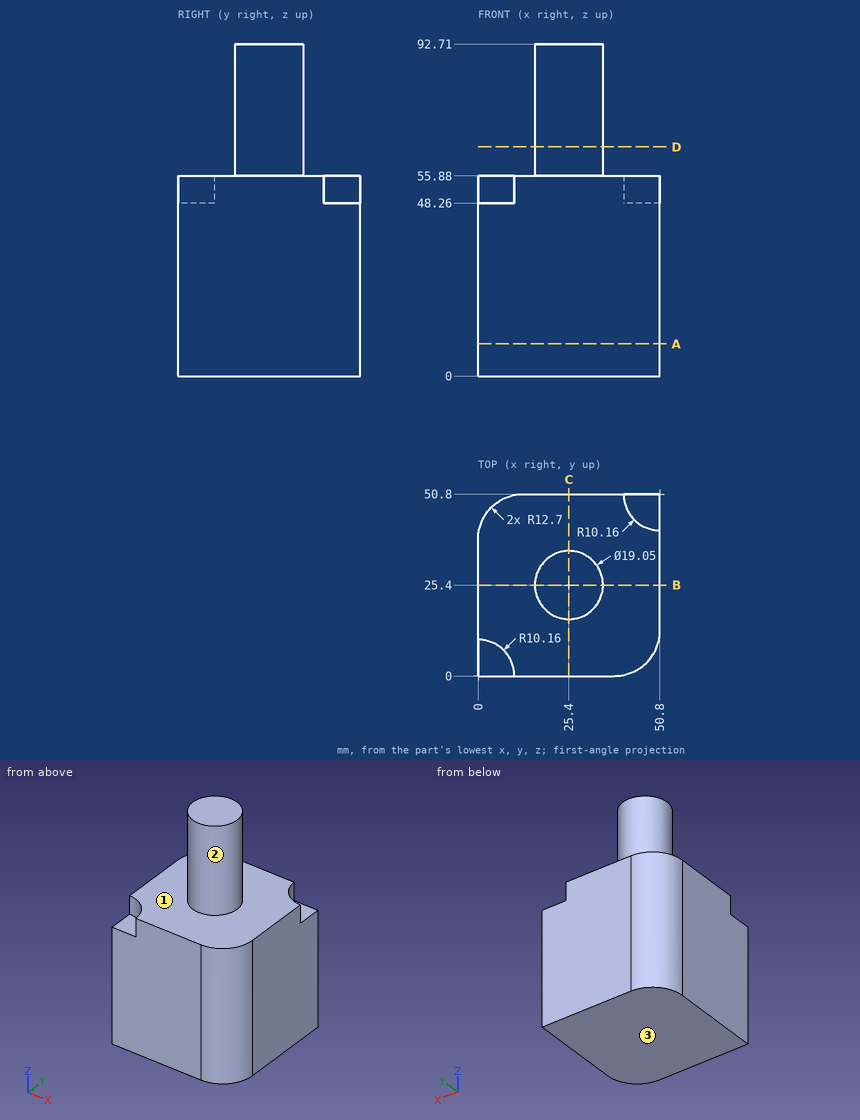
Study the drawing (mm; zero at the part's minimum x, y, z) and answer. Give positions to 0.01 mm unless a question says otherwise; leave off trailing zeros. Order: outer loops, then holes, each group sorted by start corner. A loop starts at its lowest first (then second) coordinate and runs counter-clockwise, first axis right, second up.
1. Section B-B, the plane y = 25.4 is taken. Determine the outline of the cut face in (x, z) (3 decimals), and give its area (3 significant figures).
Result sheet:
outline: (0, 0) - (50.8, 0) - (50.8, 55.88) - (34.925, 55.88) - (34.925, 92.71) - (15.875, 92.71) - (15.875, 55.88) - (0, 55.88) - close
area: 3,540 mm2
2. Section A-A, the plane z = 9 is taken. Determine the outline of the cut face in (x, y).
Result sheet:
outline: (0, 0) - (38.1, 0) arc R12.7 ccw to (50.8, 12.7) - (50.8, 50.8) - (12.7, 50.8) arc R12.7 ccw to (0, 38.1) - close
3. Section D-D, the plane z = 64 is taken. Determine the outline of the cut face in (x, y) (3 decimals).
Result sheet:
outline: circle Ø19.05 at (25.4, 25.4)
4. The mould has two halves that part along Z. Classify the marked faces 1, 2 and 3: released by +Z, released by -Z, zero draft, split by the parting line, or undercut.
Result sheet:
face 1: released by +Z
face 2: zero draft
face 3: released by -Z
5. Straight lines are drawn through the part: L1, parallel to Z at x = 3.5, y = 28.5; L2, parallel to Y at x = 45.5, z = 38; L3, parallel to X at y = 23, z = 67. For each, find the intervals that lie inside material, in ascending order.
Result sheet:
L1: z = 0 to 55.88
L2: y = 2.38 to 50.8
L3: x = 16.18 to 34.62
6. Each of these flat-tipped pins is pushed along its axis until it touches: P1, Ø3, axis at x = 7, y = 5, coming from the +Z side; P2, Ø1, axis at x = 29, y = 16.5, coming from the +Z side; P3, Ø11, axis at x = 46.5, y = 45, coming from the +Z side. Where does it stop, or does it pass through?
Result sheet:
P1: stops at z = 48.26
P2: stops at z = 92.71
P3: stops at z = 55.88
